from build123d import *

# Parameters (mm, degrees)
EXTRUDE1_DEPTH     = 2.34
SKETCH2_W          = 6.35
SKETCH2_H          = 6.35
SKETCH2_R          = 1.09
EXTRUDE2_DEPTH     = 1.47
SKETCH3_W          = 4.17
SKETCH3_H          = 4.57
SKETCH3_W_2        = 4.57
SKETCH3_H_2        = 4.17
CUT_EXTRUDE1_DEPTH = 1.32
FILLET1_R          = 0.81
SKETCH4_W          = 38.1
SKETCH4_H          = 15.88
SKETCH4_R          = 1.37
EXTRUDE3_DEPTH     = 6.55
FILLET2_R          = 3.18


with BuildPart() as part:
    # Sketch1 → Extrude1 (new body)
    with BuildSketch(Plane.XY):
        Polygon((-35.56, -6.35), (-35.56, 6.35), (-21.23, 13.03), (35.56, 13.03), (35.56, -13.03), (-21.23, -13.03), align=None)
    extrude(amount=EXTRUDE1_DEPTH)

    # Sketch2 → Extrude2 (add)
    with BuildSketch(Plane(origin=(0, 0, 0), x_dir=(-1, 0, 0), z_dir=(0, 0, -1))):
        with Locations((-32.385, 9.855)):
            Rectangle(SKETCH2_W, SKETCH2_H)
        with Locations((-32.385, 9.855)):
            Circle(SKETCH2_R, mode=Mode.SUBTRACT)
        with Locations((-32.385, -9.855)):
            Rectangle(SKETCH2_W, SKETCH2_H)
        with Locations((-32.385, -9.855)):
            Circle(SKETCH2_R, mode=Mode.SUBTRACT)
        with Locations((26.665, 0)):
            Rectangle(SKETCH2_W, SKETCH2_H)
        with Locations((26.665, 0)):
            Circle(SKETCH2_R, mode=Mode.SUBTRACT)
    extrude(amount=EXTRUDE2_DEPTH)

    # Sketch3 → Cut-Extrude1 (cut)
    with BuildSketch(Plane(origin=(0, 0, 0), x_dir=(-1, 0, 0), z_dir=(0, 0, -1))):
        with Locations((-25.395, -10.745)):
            Rectangle(SKETCH3_W, SKETCH3_H)
        with Locations((-25.395, 10.745)):
            Rectangle(SKETCH3_W, SKETCH3_H)
        with Locations((33.275, 0)):
            Rectangle(SKETCH3_W_2, SKETCH3_H_2)
    extrude(amount=-CUT_EXTRUDE1_DEPTH, mode=Mode.SUBTRACT)

    # Fillet1
    fillet1_edges = [part.edges().sort_by_distance(p)[0] for p in [
        (27.48, -8.46, 0.66),
        (23.31, -8.46, 0.66),
        (27.48, 8.46, 0.66),
        (23.31, 8.46, 0.66),
        (-30.99, -2.085, 0.66),
        (-30.99, 2.085, 0.66),
    ]]
    fillet(fillet1_edges, radius=FILLET1_R)

    # Sketch4 → Extrude3 (add)
    with BuildSketch(Plane(origin=(0, 0, 0), x_dir=(-1, 0, 0), z_dir=(0, 0, -1))):
        with Locations((-3.81, 0)):
            Rectangle(SKETCH4_W, SKETCH4_H)
        with Locations((-16.51, 0)):
            Circle(SKETCH4_R, mode=Mode.SUBTRACT)
        with Locations((8.89, 0)):
            Circle(SKETCH4_R, mode=Mode.SUBTRACT)
    extrude(amount=EXTRUDE3_DEPTH)

    # Fillet2
    fillet2_edges = [part.edges().sort_by_distance(p)[0] for p in [
        (22.86, 7.94, -3.275),
        (22.86, -7.94, -3.275),
        (-15.24, -7.94, -3.275),
        (-15.24, 7.94, -3.275),
    ]]
    fillet(fillet2_edges, radius=FILLET2_R)


solid = part.part
Here's how the part is built. I have some questions about the finished solid (model axes, mm). A direction names the side the tool comes from. Coordinates: 2 decimals unless noted, no trailing zeros. Order: outer loops, then holes, each group sorted by start corner. A loop starts at its lowest first (then second) coordinate and runs counter-clockwise, first axis right, second up. Notation, with made-up numbers: M 82.5,59 L 97.5,59 A11 cw 97.5,72 Z; hole C 44,40 d8. An arc over 180 degrees is marked long. Answer as CSV lines item,"result".
Item 1: We'd pull the mould along Y, two halves only. Please class faces 4 (the face through (-27, 3.175, -1)), 5 (the face through (32, 6.68, -1)), 6 (the face through (-29.84, 0, -1)), 7 (the face through (-27, 0, 0)): +Y half, -Y half, draft (parallel to the pull), parting line (faces both ways), or undercut.
Results found:
face 4,"+Y half"
face 5,"undercut"
face 6,"draft"
face 7,"undercut"
Item 2: Imagine slicing it at A-A on z = -5.5. Write out the boundary of the cut face in (x, y), plus the area to 3 significant figures.
Results found:
outline,"M -15.24,-4.76 A3.18 ccw -12.06,-7.94 L 19.68,-7.94 A3.18 ccw 22.86,-4.76 L 22.86,4.76 A3.18 ccw 19.68,7.94 L -12.06,7.94 A3.18 ccw -15.24,4.76 Z; hole C -8.89,0 d2.74; hole C 16.51,0 d2.74"
area,"585 mm2"
Item 3: On a 3-axis mill with a long thin cutter (end or side, diameter ignored), from which of +Z, -Z, +X, -X, +Y, -Y can I reach the whole of each face in a straight line? I mean faces 1 (the face through (31, -10, -1.47)), 2 (the face through (27.48, 11, 1)), 3 (the face through (-27.705, 0.327, -0.725)). Say none if no direction works.
Results found:
face 1,"-Z, +X, +Y, -Y"
face 2,"-Z, +Y"
face 3,"-Z"
Item 4: For pin 1 (3 mm diameter, centred on y = -8.5, z = -3, fed in from +X); pin 2 (1.7 mm diameter, centred on x = 32.385, y = 9.855, fed in from -Z); pin 3 (1 mm diameter, centred on x = -27, z = -3, fed in from -Y); pin 4 (0.7 mm diameter, centred on y = -0.5, z = -0.5, fed in from -X), each with a flat end and sliding along its axis, tell me the tip position at first contact or that it passes through.
Results found:
pin 1,"x = 21.94"
pin 2,"z = 0"
pin 3,"through"
pin 4,"x = -29.84"
Item 5: Imagine slicing it at D-D on x = 0. Write out the boundary of the cut face in (y, z), plus the area to 3 significant figures.
Results found:
outline,"M -13.03,0 L -7.94,0 L -7.94,-6.55 L 7.94,-6.55 L 7.94,0 L 13.03,0 L 13.03,2.34 L -13.03,2.34 Z"
area,"165 mm2"
Item 6: Imagine slicing it at B-B on y = 0. Write out the boundary of the cut face in (x, z) (3 decimals).
Results found:
outline,"M -35.56,1.32 L -30.99,1.32 L -30.99,0 L -29.84,0 L -29.84,-1.47 L -27.755,-1.47 L -27.755,0 L -25.575,0 L -25.575,-1.47 L -23.49,-1.47 L -23.49,0 L -15.24,0 L -15.24,-6.55 L -10.26,-6.55 L -10.26,0 L -7.52,0 L -7.52,-6.55 L 15.14,-6.55 L 15.14,0 L 17.88,0 L 17.88,-6.55 L 22.86,-6.55 L 22.86,0 L 35.56,0 L 35.56,2.34 L -35.56,2.34 Z"
Item 7: Imagine slicing it at C-C on x = 16.51. Write out the boundary of the cut face in (y, z), plus the area to 3 significant figures.
Results found:
outline,"M -13.03,0 L -7.94,0 L -7.94,-6.55 L -1.37,-6.55 L -1.37,0 L 1.37,0 L 1.37,-6.55 L 7.94,-6.55 L 7.94,0 L 13.03,0 L 13.03,2.34 L -13.03,2.34 Z"
area,"147 mm2"
Item 8: If I drill on line 1 (Z direction, x = -1, y = 10); line 2 (Y direction, x = -8.89, z = -4.75); line 3 (X direction, y = -4.75, z = -3.5), over which ranges is the centre line in solid material (lowest first)?
Results found:
line 1,"0 to 2.34"
line 2,"-7.94 to -1.37, 1.37 to 7.94"
line 3,"-15.24 to 22.86"
